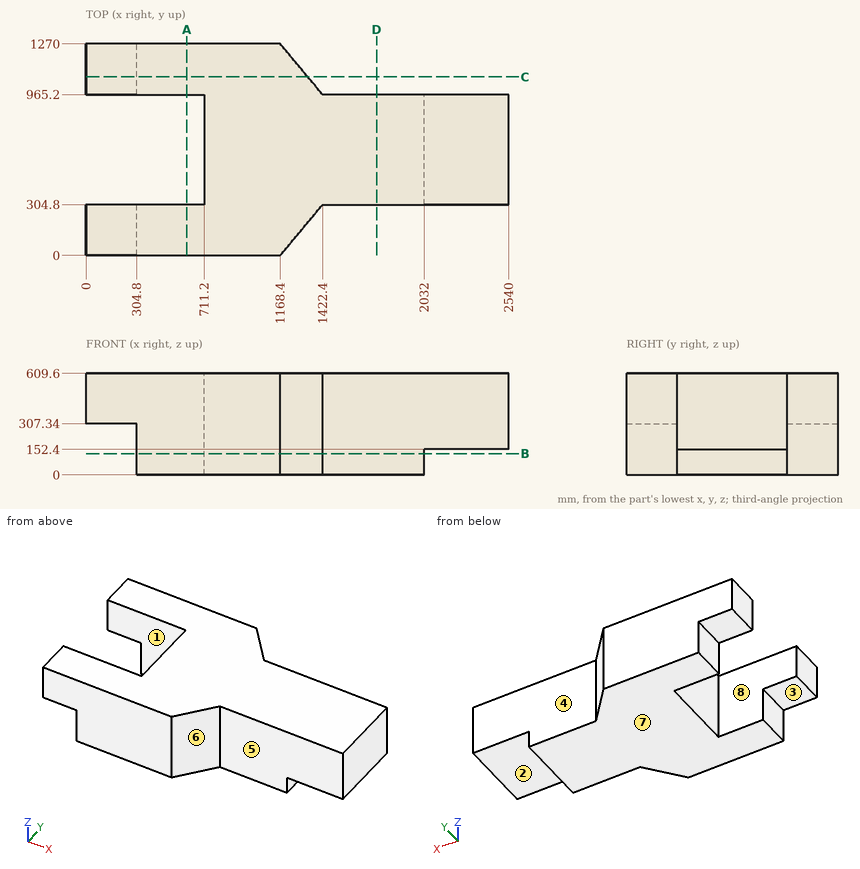
Design review of the part shown in the three views and the two pictorial views. Dimensions are in mm from the part's minimum x, y and z. A direction names the side the tool comes from. Round coordinates to 2 decimals unless told otherwise and drop trailing zeros. Loops run counter-clockwise (first coordinate to the right, second up) from the corner with the lowest first, then second, coordinate; pieces in that order, holes last. Notation, with made-up numbers: (8, 61) -> (36, 61) arc R11 ccw to (36, 74) -> close; hole circle Ø5 at (-28.5, 68.5). An arc over 180 degrees is marked (long way). Answer as a JSON object with one key per item and string values. Group by question number.
1) For the marked faces 1, 2, 3, 4 and 5, list the 3-axis set-ups (+Z, -Z, +X, -X, +Y, -Y) from which the entire face can be reached by the end or side of a thin tool; tool diameter is ignored.
2) Mouldability with a two-part tool opening along Y and no side actions: class the marked faces 6, 7 and 8 as released by +Y, released by -Y, zero draft, split by the parting line, or undercut.
3) We need section C-C on y = 1072. Write out the cut boundary in (x, z), then the cut area to 3 significant figures.
4) We need section A-A on x = 605.5. Write out the cut boundary in (y, z).
5) For pin 1 Ø2 at (x, z) = (1269.5, 407.5) entering from +Y; pin 2 Ø3 at (x, z) = (1554, 464) entering from -Y; pin 3 Ø4 at (x, z) = (1402.5, 413.5) entering from -Y, all flat-tipped, find the tip position at first contact; note any pin that passes through.
6) For line 1 (Y direction, x = 566.5, z = 494.5); line 2 (Y direction, x = 1970, z = 388); line 3 (X direction, y = 609.5, z = 108), list the stretches that pass through material, from the lowest coordinate up. Write a range as [from, to].
7) We need section B-B on z = 127. Write out the cut boundary in (x, y), then the cut area to 3 significant figures.
8) We need section D-D on x = 1747. Write out the cut boundary in (y, z), then the cut area to 3 significant figures.
Result set:
{
 "1": {"face 1": "+Z, -Z, -X", "face 2": "-Z, +X, +Y, -Y", "face 3": "-Z, -X, +Y, -Y", "face 4": "+Z, -Z, +X, +Y", "face 5": "+Z, -Z, +X, -Y"},
 "2": {"face 6": "released by -Y", "face 7": "zero draft", "face 8": "undercut"},
 "3": {"outline": "(0, 307.34) -> (304.8, 307.34) -> (304.8, 0) -> (1333.4, 0) -> (1333.4, 609.6) -> (0, 609.6) -> close", "area": "719,000 mm²"},
 "4": {"outline": "(0, 0) -> (304.8, 0) -> (304.8, 609.6) -> (0, 609.6) -> close; (965.2, 0) -> (1270, 0) -> (1270, 609.6) -> (965.2, 609.6) -> close"},
 "5": {"pin 1": "y = 1149.88", "pin 2": "y = 304.8", "pin 3": "y = 278.52"},
 "6": {"line 1": "[0, 304.8], [965.2, 1270]", "line 2": "[304.8, 965.2]", "line 3": "[711.2, 2032]"},
 "7": {"outline": "(304.8, 0) -> (1168.4, 0) -> (1422.4, 304.8) -> (2032, 304.8) -> (2032, 965.2) -> (1422.4, 965.2) -> (1168.4, 1270) -> (304.8, 1270) -> (304.8, 965.2) -> (711.2, 965.2) -> (711.2, 304.8) -> (304.8, 304.8) -> close", "area": "1,480,000 mm²"},
 "8": {"outline": "(304.8, 0) -> (965.2, 0) -> (965.2, 609.6) -> (304.8, 609.6) -> close", "area": "403,000 mm²"}
}
